CAD build for the part. Positions are in the model's coordinates, mm. A direction names the side the tool comes from. Round coordinates to 2 decimals unless told otherwise and drop trailing zeros. Write each loop counter-clockwise with the first axis right and the second up, starting at its lowest first coordinate (ties: lowest second). Pieces come first, ordered by that corner, then holes. Notation, with made-up numbers: (8.25, 72) - (48.25, 72) arc R10 cw to (48.25, 84) - close; hole circle Ø11 at (83, 17.5). An arc over 180 degrees is marked (long way). Use one line per item in the form item = value. Start each with the question number.
Item 1: Pin check, flat tips, straight feed: pin 1 (11.5 mm diameter, centred on x = -17.1, z = 13.55, fed in from +Y); pin 2 (3 mm diameter, centred on x = -17.5, y = -16, fed in from +Z); pin 3 (1 mm diameter, centred on x = 9.5, y = -3, fed in from -Z); pin 4 (7.5 mm diameter, centred on x = 12, y = -0.5, fed in from +Z). Stop position of each tip, or through.
Item 2: Band-saw the part on A-A, the plane z = 7.5. List the corners of the cut face in (x, y), and give its area (3 significant figures).
Item 3: Band-saw the part on C-C, the plane y = -4.5. List the corners of the cut face in (x, z), and give its area (3 significant figures).
Item 4: Drill centre lines: L1, parallel to Y at x = 26, z = 11; L2, parallel to Z at x = -17.1, y = 21; L3, parallel to X at y = -19, z = 24. Where is each one in solid material? Low to high.
Item 5: Pull direction X, two halves, no side cores. Call faces 6 (the flat face through (0, 22.9, 13)), 7 (the cylindrical face through (28.06, 9.72, 29.07)), 8 (the flat face through (0, 20.5, 12)): +X half, -X half, draft (parallel to the pull), parting line (faces both ways), or undercut.
Item 6: Band-saw the part on D-D, the plane z = 13.55. List the corners of the cut face in (x, y), and give its area (3 significant figures).
Item 7: Tool access for faces 1 (the flat face through (14, 5, 25.2)), 2 (the flat face through (-32, 0, 13)), 3 (the flat face through (0, -20.5, 12)), 4 (the flat face through (0, -22.9, 13)), 5 (the cylindrical face through (-21.87, 21.72, 15.05)): list every direction of +Z, -Z, +X, -X, +Y, -Y with a clear straight run to the whole face (end or side of a thin tool).
Item 8: Band-saw the part on B-B, the plane x = -9. List the corners of the cut face in (y, z).
from build123d import *

# Parameters (mm, degrees)
F4_W      = 64
F4_H      = 45.8
F4_W_2    = 59.2
F4_H_2    = 41
F5_DEPTH  = 24.7
F6_W      = 64
F6_H      = 45.8
F6_W_2    = 59.2
F6_H_2    = 41
F7_DEPTH  = 2.4
F8_R      = 5
F9_DEPTH  = 1.9
F10_R     = 14.82
F10_R_2   = 12.42
F11_DEPTH = 4
F12_DEPTH = 1.9
F13_R     = 5
F14_DEPTH = 2.4


with BuildPart() as f5:
    # F4 (on Top) → F5 (new body)
    with BuildSketch(Plane.XY):
        Rectangle(F4_W, F4_H)
        Rectangle(F4_W_2, F4_H_2, mode=Mode.SUBTRACT)
    extrude(amount=F5_DEPTH)

    # F6 (on face) → F7 (join)
    with BuildSketch(Plane.XY.offset(24.7)):
        Rectangle(F6_W, F6_H)
        Rectangle(F6_W_2, F6_H_2, mode=Mode.SUBTRACT)
        Rectangle(F6_W_2, F6_H_2)
    extrude(amount=F7_DEPTH)

    # F8 (on face) → F9 (cut)
    with BuildSketch(Plane.XY.offset(27.1)):
        with Locations((-18.6, 7.5)):
            Circle(F8_R)
    extrude(amount=-F9_DEPTH, mode=Mode.SUBTRACT)

    # F10 (on face) → F11 (join)
    with BuildSketch(Plane.XY.offset(27.1)):
        with Locations((13.926, 5.264)):
            Circle(F10_R)
        with Locations((13.926, 5.264)):
            Circle(F10_R_2, mode=Mode.SUBTRACT)
    extrude(amount=F11_DEPTH)

    # F12 (cut): a face of the model
    f12_faces = [f5.faces().sort_by_distance(p)[0] for p in [
        (13.926, 5.264, 27.1),
    ]]
    extrude(f12_faces, amount=-F12_DEPTH, mode=Mode.SUBTRACT)

    # F13 (on face) → F14 (cut)
    with BuildSketch(Plane(origin=(0, 22.9, 0), x_dir=(-1, 0, 0), z_dir=(0, 1, 0))):
        with Locations((17.1, 13.55)):
            Circle(F13_R)
    extrude(amount=-F14_DEPTH, mode=Mode.SUBTRACT)


solid = f5.part
Determined:
q1.pin_1 = 22.9
q1.pin_2 = 27.1
q1.pin_3 = 24.7
q1.pin_4 = 25.2
q2.outline = (-32, -22.9) - (32, -22.9) - (32, 22.9) - (-32, 22.9) - close; hole (-29.6, -20.5) - (29.6, -20.5) - (29.6, 20.5) - (-29.6, 20.5) - close
q2.area = 504 mm²
q3.outline = (-32, 0) - (-29.6, 0) - (-29.6, 24.7) - (29.6, 24.7) - (29.6, 0) - (32, 0) - (32, 27.1) - (25.07, 27.1) - (25.07, 31.1) - (21.6, 31.1) - (21.6, 25.2) - (6.25, 25.2) - (6.25, 31.1) - (2.78, 31.1) - (2.78, 27.1) - (-32, 27.1) - close
q3.area = 271 mm²
q4.L1 = -22.9 to -20.5, 20.5 to 22.9
q4.L2 = 0 to 8.55, 18.55 to 27.1
q4.L3 = -32 to -29.6, 29.6 to 32
q5.face_6 = draft
q5.face_7 = parting line
q5.face_8 = undercut
q6.outline = (-32, -22.9) - (32, -22.9) - (32, 22.9) - (-12.1, 22.9) - (-12.1, 20.5) - (29.6, 20.5) - (29.6, -20.5) - (-29.6, -20.5) - (-29.6, 20.5) - (-22.1, 20.5) - (-22.1, 22.9) - (-32, 22.9) - close
q6.area = 480 mm²
q7.face_1 = +Z
q7.face_2 = +Z, -Z, -X, +Y, -Y
q7.face_3 = -Z
q7.face_4 = +Z, -Z, +X, -X, -Y
q7.face_5 = +Y
q8.outline = (-22.9, 0) - (-20.5, 0) - (-20.5, 24.7) - (20.5, 24.7) - (20.5, 0) - (22.9, 0) - (22.9, 27.1) - (-22.9, 27.1) - close
